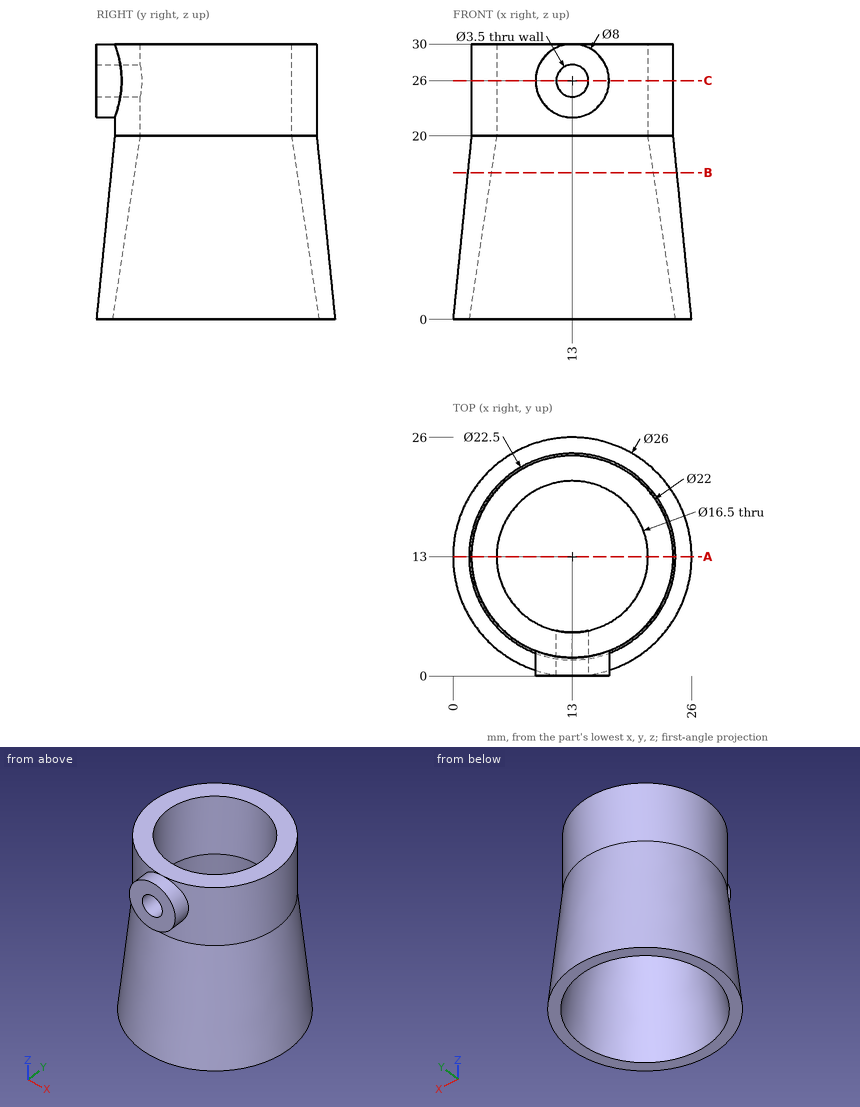
Geometry: see drawing. Coordinates: mm, zero at the bounding-box minimum. Coordinates: 2 decimals unless noted, no trailing zeros. Write each loop counter-clockwise with the first axis right and the second up, starting at its lowest first coordinate (ties: lowest second). Pieces come first, ordered by that corner, then holes. Notation, with made-up numbers: (48.5, 44.25) - (66.5, 44.25) arc R11 ccw to (66.5, 50.25) - close; hole circle Ø8 at (27, 14.5). An arc over 180 degrees is marked (long way). Put each result on its own line as item: value. Start each with the question number.
1) Ray query, L1, parallel to X at y = 1.35, z = 26; L2, parallel to X at y = 10.75, z = 19; L3, parallel to Y at x = 7.75, z = 20. Return the intervals inside material, ascending.
2) Cut plane C-C (z = 26). Return the cut outline in (x, y), plus the area to 3 significant figures.
3) Contact query for flat-ended pins moving along their axis: pin 1 (8 mm diameter, centred on y = 14.5, z = 17.5, fed in from +X); pin 2 (5 mm diameter, centred on y = 3, z = 19.5, fed in from +X); pin 3 (8 mm diameter, centred on y = 15, z = 8, fed in from +X). Output: stop coordinate, or through.
4) Cut plane A-A (y = 13). Return the cut outline in (x, z), plus the area to 3 significant figures.
5) Cut plane B-B (z = 16). Return the cut outline in (x, y).
Resolved:
1. L1: x = 9 to 11.25, 14.75 to 17
1. L2: x = 2.13 to 4.91, 21.09 to 23.87
1. L3: y = 3.33 to 6.64, 19.36 to 22.67
2. outline: (9, 0) - (11.25, 0) - (11.25, 4.94) arc R8.25 cw (long way) to (14.75, 4.94) - (14.75, 0) - (17, 0) - (17, 2.75) arc R11 ccw (long way) to (9, 2.75) - close
2. area: 167 mm2
3. pin 1: stops at x = 24.63
3. pin 2: stops at x = 21.14
3. pin 3: stops at x = 25.56
4. outline: (0, 0) - (1.75, 0) - (4.75, 20) - (4.75, 30) - (2, 30) - (2, 20) - close; (21.25, 20) - (24.25, 0) - (26, 0) - (24, 20) - (24, 30) - (21.25, 30) - close
4. area: 145 mm2
5. outline: circle Ø22.8 at (13, 13); hole circle Ø17.7 at (13, 13)
